Input: dimensioned drawing with shaded views. Units: mm. Origin: part minimum x, y, z. A direction names the side the tool comes from. Round coordinates to 2 decimals unless told otherwise and drop trailing zeros. Loops run counter-clockwise (first coordinate to the right, second up) from the corner with the lowest first, then second, coordinate; pieces in that order, holes last. Notation, with made-up numbers: (88, 1.25) - (129, 1.25) arc R20 cw to (129, 28.25) - close; hole circle Ø9 at (48.25, 89.25). An arc over 180 degrees is marked (long way). Answer as a JSON object with one key per item and string values. Group by question number.
Item 1: Reachability of the marked faces 4 and 5 from +Z, -Z, +X, -X, +Y, -Y: full face, straight path, thin tool, end or side. Return the list, or none.
Item 2: Section A-A (y = 16). Return the cut outline in (x, z), plus the area to 3 significant figures.
Item 3: Draft query along Y for the marked faces 1, 2 and 3. Return one class per face: released by +Y, released by -Y, zero draft, split by the parting line, or undercut.
Item 4: First-contact query: pin 1 (2 mm diameter, centred on x = 3.5, y = 19, fed in from -Z); pin 2 (7 mm diameter, centred on y = 16, z = 16, fed in from -X); pin 3 (16 mm diameter, centred on y = 22.5, z = 9, fed in from +X); pin 4 (2 mm diameter, centred on x = 1, z = 14, fed in from +Y). Flat tips, straight axial feed; report the tip coordinate or a pass-through.
Item 5: Line query: line 1 (Y direction, x = 2.95, z = 16); line 2 (Y direction, x = 2.7, z = 11); line 3 (Z direction, x = 2.05, y = 9) (1 decimal). Output: solid intervals per line, ascending.
Item 6: Section C-C (x = 3.55). Return the cut outline in (y, z).
Item 7: Section D-D (y = 24.5). Return the cut outline in (x, z).
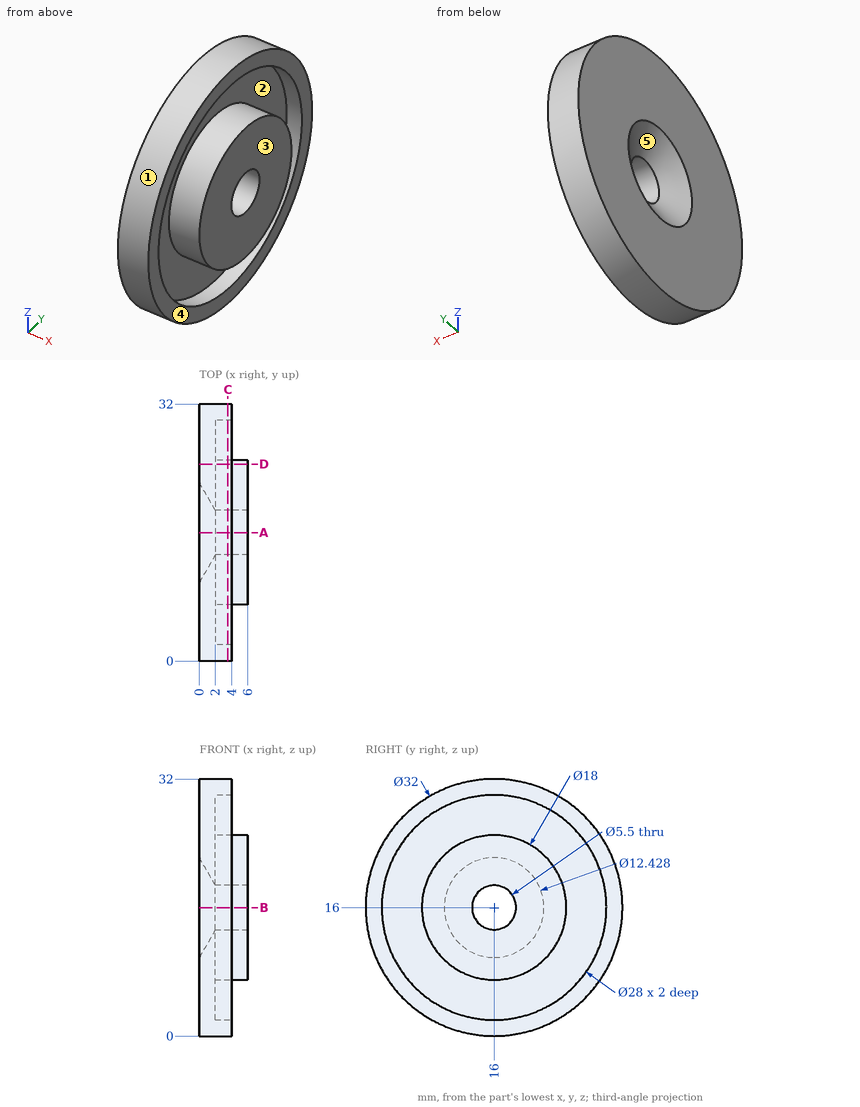
Values:
{
 "1": {"face 4": "+X", "face 5": "-X"},
 "2": {"outline": "(0, 0) - (4, 0) - (4, 2) - (2, 2) - (2, 7) - (6, 7) - (6, 13.25) - (2, 13.25) - (0, 9.79) - close; (0, 22.21) - (2, 18.75) - (6, 18.75) - (6, 25) - (2, 25) - (2, 30) - (4, 30) - (4, 32) - (0, 32) - close", "area": "104 mm^2"},
 "3": {"face 1": "split by the parting line", "face 2": "undercut", "face 3": "zero draft"},
 "4": {"pin 1": "stops at z = 0.13", "pin 2": "stops at x = 1.57", "pin 3": "stops at x = 6", "pin 4": "stops at y = 31.97"},
 "5": {"line 1": "y = 0 to 2, 7 to 13.25, 18.75 to 25, 30 to 32", "line 2": "y = 0.8 to 2.92, 8.52 to 23.48, 29.08 to 31.2", "line 3": "z = 1.6 to 3.9, 10.3 to 21.7, 28.1 to 30.4"},
 "6": {"outline": "circle Ø32 at (16, 16); circle Ø18 at (16, 16); hole circle Ø28 at (16, 16); hole circle Ø5.5 at (16, 16)"},
 "7": {"outline": "(0, 2.44) - (4, 2.44) - (4, 4.88) - (2, 4.88) - (2, 13.04) - (6, 13.04) - (6, 18.96) - (2, 18.96) - (2, 27.12) - (4, 27.12) - (4, 29.56) - (0, 29.56) - close"}
}
